Input: part model. Units: mm. Frame: model coordinates. A direction names the side the tool comes from. Coordinates: 2 decimals unless noted, no trailing zeros. Order: outer loops, then holes, each group sorted by start corner. A loop starts at its lowest first (then second) coordinate and runs counter-clockwise, first axis right, second up. Notation, with made-up numbers: (17.5, 65.25) - (72.5, 65.25) arc R22 cw to (72.5, 103.25) - close; hole circle Ø2 at (25, 44.25). An arc over 180 degrees is marked (long way). Use a Markdown table: item, result. Add a question column.
from build123d import *

# Parameters (mm, degrees)
IZIM2_R                     = 34.224414592
IZIM2_R_2                   = 29.224414592
IZIM2_R_3                   = 2.396512678
Y_KSEKLIK_EKSTR_ZYON6_DEPTH = 3
IZIM2_3_R                   = 2.396512678
Y_KSEKLIK_EKSTR_ZYON7_DEPTH = 30


with BuildPart() as part:
    # izim2 → Y_kseklik-Ekstr_zyon6 (new body)
    with BuildSketch(Plane(origin=(0, 0, 0), x_dir=(1, 0, 0), z_dir=(0, 1, 0))):
        Circle(IZIM2_R)
        Circle(IZIM2_R_2, mode=Mode.SUBTRACT)
        with Locations((0, -29.224414592)):
            Circle(IZIM2_R_3, mode=Mode.SUBTRACT)
        with Locations((-29.224414592, 0)):
            Circle(IZIM2_R_3, mode=Mode.SUBTRACT)
        with Locations((0, 29.224414592)):
            Circle(IZIM2_R_3, mode=Mode.SUBTRACT)
        with Locations((29.224414592, 0)):
            Circle(IZIM2_R_3, mode=Mode.SUBTRACT)
        with Locations((0, -29.224414592)):
            Circle(IZIM2_R_3)
        Circle(IZIM2_R_2)
        with Locations((29.224414592, 0)):
            Circle(IZIM2_R_3)
        with Locations((0, 29.224414592)):
            Circle(IZIM2_R_3)
        with Locations((-29.224414592, 0)):
            Circle(IZIM2_R_3)
    extrude(amount=Y_KSEKLIK_EKSTR_ZYON6_DEPTH)

    # izim2_3 → Y_kseklik-Ekstr_zyon7 (add)
    with BuildSketch(Plane(origin=(0, 0, 0), x_dir=(1, 0, 0), z_dir=(0, 1, 0))):
        with Locations((0, 29.224414592)):
            Circle(IZIM2_3_R)
        with Locations((0, -29.224414592)):
            Circle(IZIM2_3_R)
        with Locations((-29.224414592, 0)):
            Circle(IZIM2_3_R)
        with Locations((29.224414592, 0)):
            Circle(IZIM2_3_R)
    extrude(amount=-Y_KSEKLIK_EKSTR_ZYON7_DEPTH)


solid = part.part
1) Cut plane C-C (y = -4.5). Return the cut outline in (x, z), and give its area (3 significant figures).
2) Cut plane A-A (z = 0). Return the cut outline in (x, y), and give its area (3 significant figures).
3) Material intervals for L1, parallel to Y at x = -6, z = -23; L2, parallel to X at y = -26.5, z = 27.5; L3, parallel to X at y = -5, z = 1, sorted ascending.
4) Reachability of faces 4 (the cylindrical face through (-31.62, -14.79, -0.11)), 5 (the flat face through (0, 3, 0)) from +Z, -Z, +X, -X, +Y, -Y: full face, straight path, thin tool, end or side. Return the list, or none.
5) Cut plane D-D (x = -25). Return the cut outline in (y, z), and give its area (3 significant figures).
6) Contact query for flat-ended pins moving along their axis: P1, Ø5, axis at x = -17.5, z = -8.5, coming from the -Y side; P2, Ø8, axis at x = -1, y = -20.5, coming from the -Z side; P3, Ø10, axis at y = -3, z = -16, coming from the -X side. Output: stop coordinate, or through.
7) Pull-direction query (Z, two-part tool) for faces 1 (the cylindrical face through (-0.31, -14.79, 26.85)), 2 (the flat face through (29, -30, 0)), 3 (the cylindrical face through (32.644, 1.479, -10.28)); classes: pulls with the +Z half, pulls with the -Z half, needs draft (parallel to the pull), parting line crosses it, or undercut.
8) Cut plane B-B (x = 0). Return the cut outline in (y, z).
Computed:
| question | item | result |
|---|---|---|
| 1 | outline | circle Ø4.79 at (-29.22, 0); circle Ø4.79 at (0, -29.22); circle Ø4.79 at (0, 29.22); circle Ø4.79 at (29.22, 0) |
| 1 | area | 72.2 mm2 |
| 2 | outline | (-34.22, 0) - (-31.62, 0) - (-31.62, -30) - (-26.83, -30) - (-26.83, 0) - (26.83, 0) - (26.83, -30) - (31.62, -30) - (31.62, 0) - (34.22, 0) - (34.22, 3) - (-34.22, 3) - close |
| 2 | area | 493 mm2 |
| 3 | L1 | y = 0 to 3 |
| 3 | L2 | x = -1.66 to 1.66 |
| 3 | L3 | x = -31.4 to -27.05, 27.05 to 31.4 |
| 4 | face 4 | -Y |
| 4 | face 5 | +Z, -Z, +X, -X, +Y |
| 5 | outline | (0, -23.37) - (3, -23.37) - (3, 23.37) - (0, 23.37) - close |
| 5 | area | 140 mm2 |
| 6 | P1 | stops at y = 0 |
| 6 | P2 | stops at z = -31.62 |
| 6 | P3 | stops at x = -32.05 |
| 7 | face 1 | undercut |
| 7 | face 2 | needs draft |
| 7 | face 3 | parting line crosses it |
| 8 | outline | (-30, -31.62) - (0, -31.62) - (0, -34.22) - (3, -34.22) - (3, 34.22) - (0, 34.22) - (0, 31.62) - (-30, 31.62) - (-30, 26.83) - (0, 26.83) - (0, -26.83) - (-30, -26.83) - close |
